Part print with two shaded views. Sizes in mm from the minimum x, y, z corner. A direction names the side the tool comes from. Round coordinates to 2 decimals unless told otherwise and drop trailing zeros. Order: outer loops, then holes, each group sorted by start corner. A loop starts at its lowest first (then second) coordinate and runs counter-clockwise, first axis right, second up. Notation, with made-up numbers: M 44,70.25 L 74,70.25 A20 cw 74,84.25 Z; hole C 48,4.25 d10. An arc over 180 degrees is marked long. Answer as a JSON object with one key per item and string values.
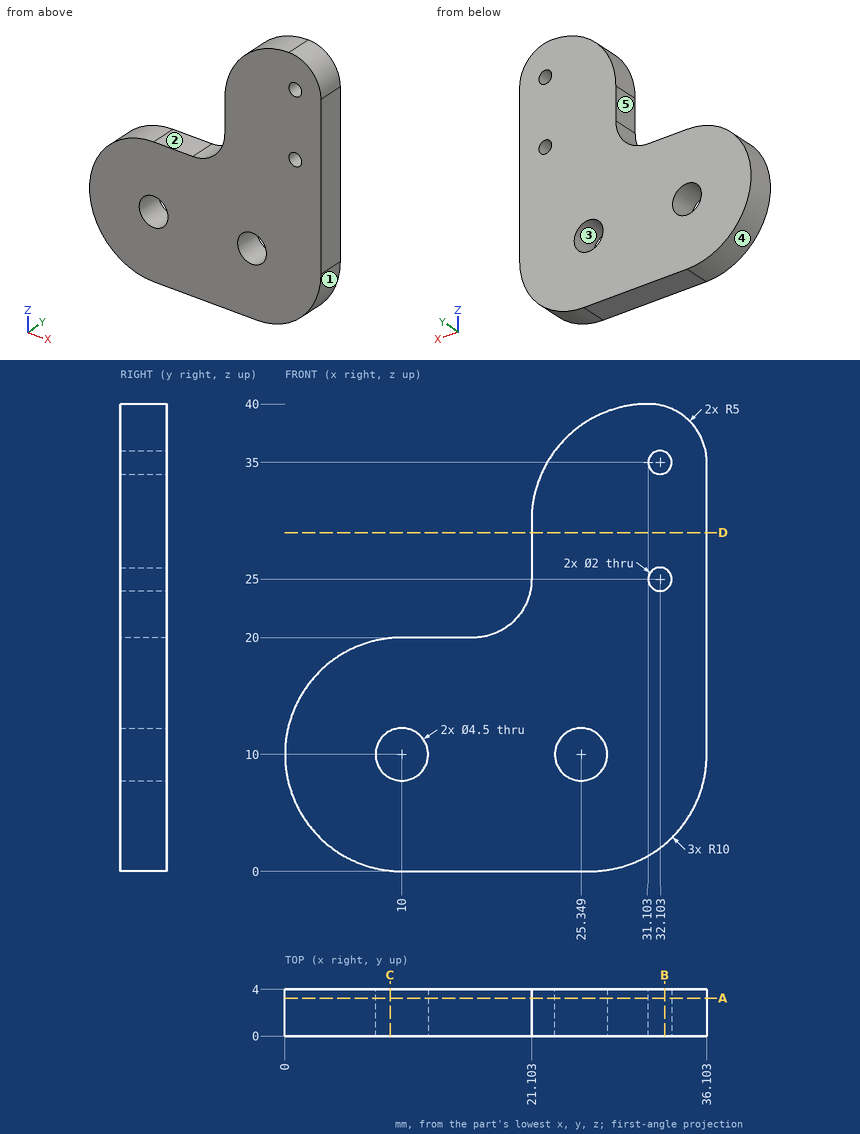
Item 1: Saw through at A-A on y = 3.25. List the corners of the cut face in (x, z).
Worked answers:
{"outline": "M 10,0 L 26.1,0 A10 ccw 36.1,10 L 36.1,35 A5 ccw 31.1,40 A10 ccw 21.1,30 L 21.1,25 A5 cw 16.1,20 L 10,20 A10 ccw Z; hole C 10,10 d4.5; hole C 25.35,10 d4.5; hole C 32.1,25 d2; hole C 32.1,35 d2"}
Item 2: 3-axis set-ups, long thin cutter, end or side, ignore diameter. For the marked faces 4 and 5: which of +Z, -Z, +X, -X, +Y, -Y reach the whole face in a straight line?
Worked answers:
{"face 4": "-X, +Y, -Y", "face 5": "+Z, -X, +Y, -Y"}
Item 3: Saw through at B-B on x = 32.5. List the corners of the cut face in (y, z).
Worked answers:
{"outline": "M 0,2.31 L 4,2.31 L 4,24.08 L 0,24.08 Z; M 0,25.92 L 4,25.92 L 4,34.08 L 0,34.08 Z; M 0,35.92 L 4,35.92 L 4,39.8 L 0,39.8 Z"}
Item 4: Drop flat-ended pins along their axis: pin 1 Ø1.2 at (y, z) = (1.5, 28.5) entering from -X; pin 2 Ø1 at (y, z) = (2, 23) entering from -X; pin 3 Ø1.5 at (y, z) = (2.5, 4) entering from +X. Give the stop position or say it passes through.
Worked answers:
{"pin 1": "stops at x = 21.1", "pin 2": "stops at x = 20.43", "pin 3": "stops at x = 34.61"}
Item 5: Saw through at D-D on z = 29. List the corners of the cut face in (x, y), and give its area (3 significant figures).
Worked answers:
{"outline": "M 21.1,0 L 36.1,0 L 36.1,4 L 21.1,4 Z", "area": "60.0 mm2"}
Item 6: Two-plate mould, pull along Z, no slides. Class the marked faces 1, 2 and 3: released by +Z, released by -Z, zero draft, split by the parting line, or undercut.
Worked answers:
{"face 1": "released by -Z", "face 2": "released by +Z", "face 3": "undercut"}
Item 7: Saw through at C-C on x = 9. List the corners of the cut face in (y, z).
Worked answers:
{"outline": "M 0,0.05 L 4,0.05 L 4,7.98 L 0,7.98 Z; M 0,12.02 L 4,12.02 L 4,19.95 L 0,19.95 Z"}
Item 8: Wall check: line 1 along Z through (x, y) = (10, 2.85); line 2 along X through (y, z) = (2.35, 10.5) (1 decimal); line 3 along Z through (x, y) = (26.5, 3.4). Give the ranges that are in metal, low to high. Write a range as [from, to].
Worked answers:
{"line 1": "z = [0, 7.75], [12.25, 20]", "line 2": "x = [0, 7.8], [12.2, 23.2], [27.5, 36.1]", "line 3": "z = [0.01, 8.07], [11.93, 38.88]"}
